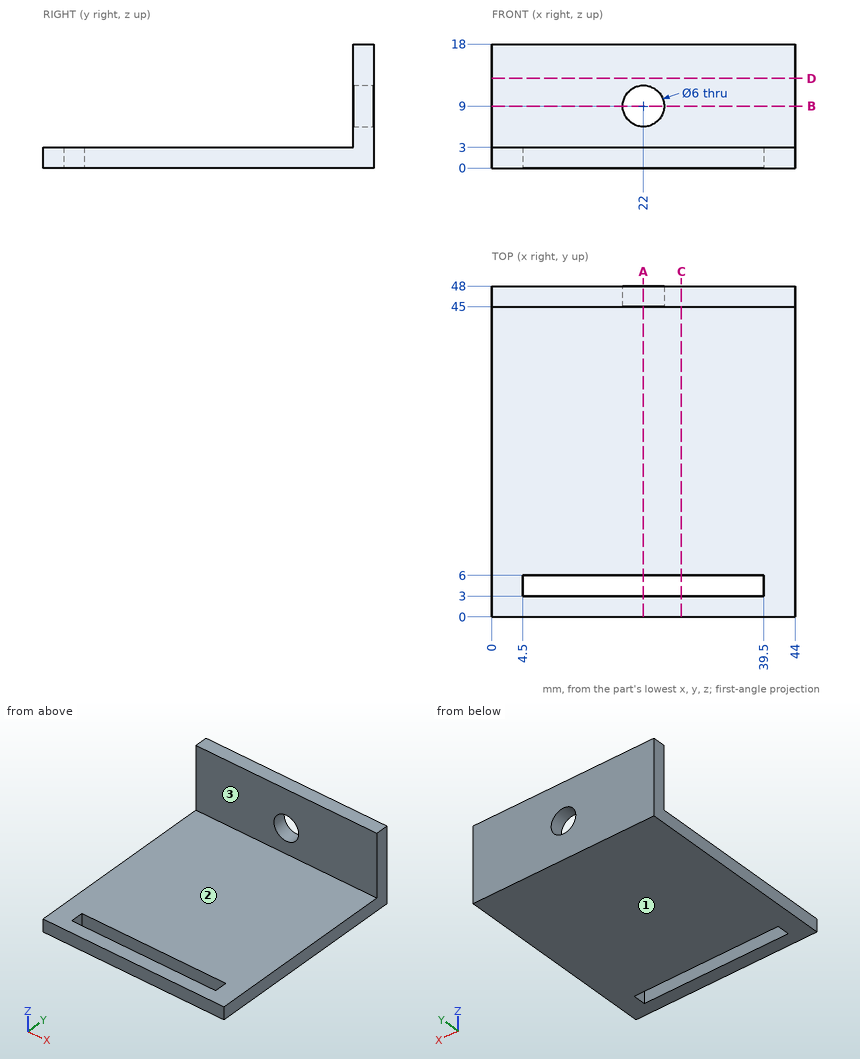
Study the drawing (mm; zero at the part's minimum x, y, z) and answer. Give positions to 0.01 mm unless a question says otherwise; leave off trailing zeros. Order: outer loops, then holes, each group sorted by start corner. A loop starts at its lowest first (then second) coordinate and runs counter-clockwise, first axis right, second up.
1. This flat-tipped pin is pushed along its axis until it touches: P1, Ø4.5, axis at x = 14.5, z = 8.5, coming from the -Y side. Where does it stop, or does it pass through?
Result sheet:
P1: stops at y = 45
2. Section D-D, the plane z = 13 is taken. Determine the outline of the cut face in (x, y), and give its area (3 significant figures).
Result sheet:
outline: (0, 45) - (44, 45) - (44, 48) - (0, 48) - close
area: 132 mm2
3. Section B-B, the plane z = 9 is taken. Determine the outline of the cut face in (x, y).
Result sheet:
outline: (0, 45) - (19, 45) - (19, 48) - (0, 48) - close; (25, 45) - (44, 45) - (44, 48) - (25, 48) - close
4. Section C-C, the plane x = 27.5 is taken. Determine the outline of the cut face in (y, z).
Result sheet:
outline: (0, 0) - (3, 0) - (3, 3) - (0, 3) - close; (6, 0) - (48, 0) - (48, 18) - (45, 18) - (45, 3) - (6, 3) - close
5. Straight lines are drawn through the part: L1, parallel to Z at x = 22, y = 47.1; L2, parallel to X at y = 45.8, z = 9; L3, parallel to Y at x = 19, z = 1.5. For each, find the intervals that lie inside material, in ascending order.
Result sheet:
L1: z = 0 to 6, 12 to 18
L2: x = 0 to 19, 25 to 44
L3: y = 0 to 3, 6 to 48
6. Section A-A, the plane x = 22 is taken. Determine the outline of the cut face in (y, z).
Result sheet:
outline: (0, 0) - (3, 0) - (3, 3) - (0, 3) - close; (6, 0) - (48, 0) - (48, 6) - (45, 6) - (45, 3) - (6, 3) - close; (45, 12) - (48, 12) - (48, 18) - (45, 18) - close
7. The mould has two halves that part along Z. Classify the marked faces 1, 2 and 3: released by +Z, released by -Z, zero draft, split by the parting line, or undercut.
Result sheet:
face 1: released by -Z
face 2: released by +Z
face 3: zero draft
